Model file for the job. Use its own axes, mm. Face numbers are marked on the shaded views. A direction names the side the tool comes from. Round coordinates to 2 decimals unless told otherwise and drop trailing zeros. Loops run counter-clockwise (first coordinate to the right, second up) from the corner with the lowest first, then second, coordinate; pieces in that order, holes last. Notation, with made-up numbers: (-34.75, -19.75) - (23.25, -19.75) arc R11 ccw to (23.25, -1.75) - close; hole circle Ø5 at (31, 82.5). An arc over 180 degrees is marked (long way). Answer as a JSON object with one key per item and string values.
from build123d import *

# Parameters (mm, degrees)
BOSS_EXTRUDE1_DEPTH = 65
SKETCH1_W           = 50
SKETCH1_H           = 50
BOSS_EXTRUDE2_DEPTH = 35
SKETCH3_R           = 13
CUT_EXTRUDE1_DEPTH  = 70


with BuildPart() as part:
    # Sketch2 → Boss-Extrude1 (new body, symmetric)
    with BuildSketch(Plane.XY):
        Polygon((0, -25), (17.67766953, -17.67766953), (25, 0), (17.67766953, 17.67766953), (0, 25), (-17.67766953, 17.67766953), (-25, 0), (-17.67766953, -17.67766953), align=None)
    extrude(amount=BOSS_EXTRUDE1_DEPTH, both=True)

    # Sketch1 → Boss-Extrude2 (add, symmetric)
    with BuildSketch(Plane.XY):
        Rectangle(SKETCH1_W, SKETCH1_H)
    extrude(amount=BOSS_EXTRUDE2_DEPTH, both=True)

    # Sketch3 → Cut-Extrude1 (cut)
    with BuildSketch(Plane(origin=(25, 0, 0), x_dir=(0, 0, -1), z_dir=(1, 0, 0))):
        Circle(SKETCH3_R)
    extrude(amount=-CUT_EXTRUDE1_DEPTH, mode=Mode.SUBTRACT)


solid = part.part
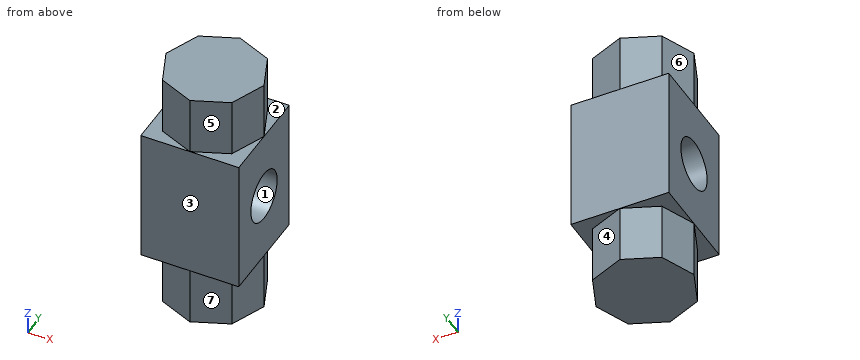
1) Drop a flat-ended pin along its axis: P1, Ø15.5, axis at y = 0, z = 0, coming from the +X side. Give the stop position or say it passes through.
Values follow:
{"P1": "through"}
2) Two-plate mould, pull along Z, no slides. Class the marked faces 1, 2 and 3: pulls with the +Z half, pulls with the -Z half, needs draft (parallel to the pull), parting line crosses it, or undercut.
Values follow:
{"face 1": "undercut", "face 2": "pulls with the +Z half", "face 3": "needs draft"}
3) Probe probe 1 along Y at (x, z) = (7.5, 0); probe 2 along Z at (x, y) = (17.5, 11.5); probe 3 along Y at (x, z) = (8.5, -3). List the from-to ranges inside material, lowest first.
Values follow:
{"probe 1": "-25 to -13, 13 to 25", "probe 2": "-65 to -6.06, 6.06 to 65", "probe 3": "-25 to -12.65, 12.65 to 25"}
4) Slice it at B-B on y = -1.5. List the corners of the cut face in (x, z), then the cut area to 3 significant figures.
Values follow:
{"outline": "(-25, -35) - (-24.38, -35) - (-24.38, -65) - (24.38, -65) - (24.38, -35) - (25, -35) - (25, -12.91) - (-25, -12.91) - close; (-25, 12.91) - (25, 12.91) - (25, 35) - (24.38, 35) - (24.38, 65) - (-24.38, 65) - (-24.38, 35) - (-25, 35) - close", "area": "5,130 mm²"}
5) Slice it at C-C on x = 11.5. List the corners of the cut face in (y, z).
Values follow:
{"outline": "(-25, -35) - (-20.24, -35) - (-20.24, -65) - (20.24, -65) - (20.24, -35) - (25, -35) - (25, 35) - (20.24, 35) - (20.24, 65) - (-20.24, 65) - (-20.24, 35) - (-25, 35) - close; hole circle Ø26 at (0, 0)"}
6) Slice it at D-D on z = 55.5. List the corners of the cut face in (x, y).
Values follow:
{"outline": "(-25, 0) - (-17.68, -17.68) - (0, -25) - (17.68, -17.68) - (25, 0) - (17.68, 17.68) - (0, 25) - (-17.68, 17.68) - close"}
7) Slice it at A-A on z = 0. List the corners of the cut face in (x, y), then the cut area to 3 significant figures.
Values follow:
{"outline": "(-25, -25) - (25, -25) - (25, -13) - (-25, -13) - close; (-25, 13) - (25, 13) - (25, 25) - (-25, 25) - close", "area": "1,200 mm²"}
8) Tool access for the marked faces 4, 5, 6 and 7: list every direction of +Z, -Z, +X, -X, +Y, -Y with a clear straight run to the whole face (end or side of a thin tool).
Values follow:
{"face 4": "-Z, +X, +Y", "face 5": "+Z, +X, -Y", "face 6": "+Z, -X, +Y", "face 7": "-Z, +X, -Y"}
